For this review, use the dimensioned drawing (mm, ordinates from the lowest corner) and the shaded views. A direction names the side the tool comes from. Coordinates: 2 decimals unless noted, no trailing zeros. Order: outer loops, then holes, each group sorted by start corner. A loop starts at its lowest first (then second) coordinate and runs counter-clockwise, first axis right, second up. Notation, with made-up numbers: M 62.25,-4 L 88.25,-4 A12 cw 88.25,18 Z; hole C -36.5,-5.5 d1. An arc over 180 degrees is marked long. Use CSV: the item, a comma, the result in double quotes.
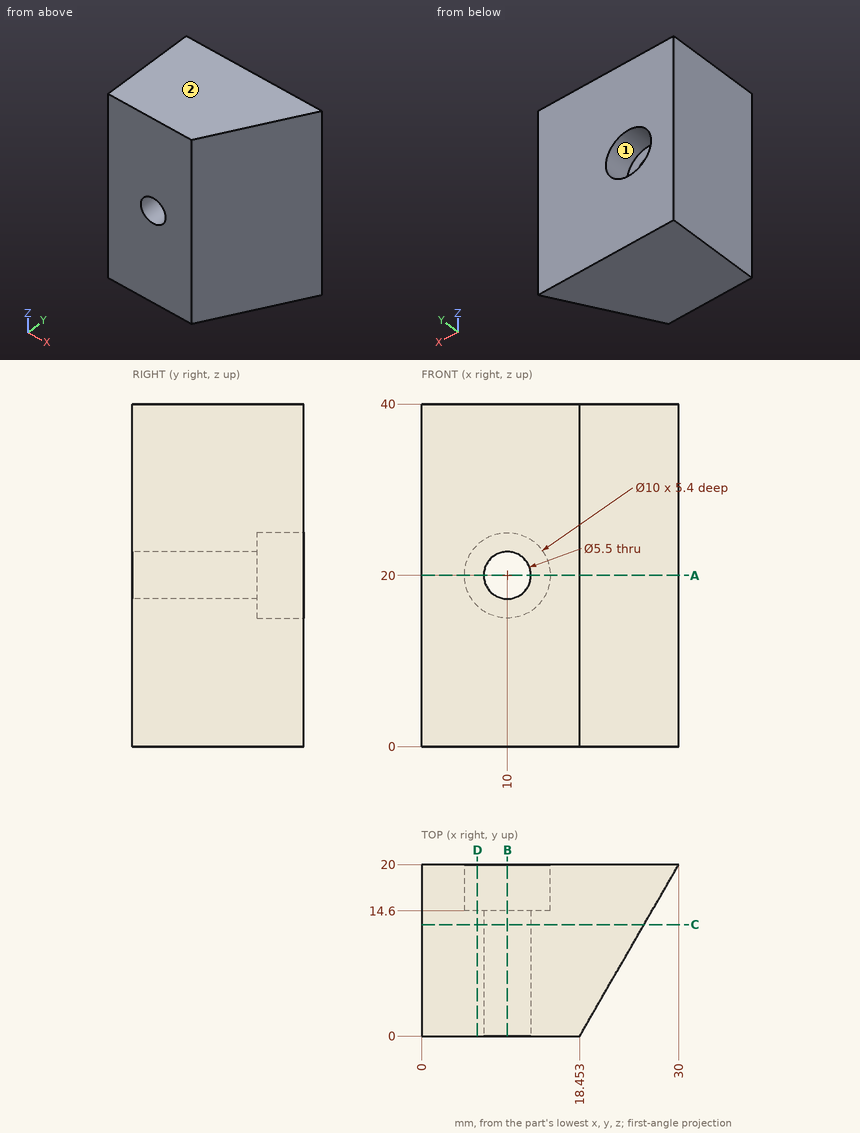
Item 1: Clearance check with flat-ended pins moving along their axes: pin 1 Ø3 at (y, z) = (8, 21.5) entering from +X; pin 2 Ø9 at (x, z) = (10, 20) entering from +Y. State where each tip first meets the part, or that it passes through.
Solutions:
pin 1,"x = 23.94"
pin 2,"y = 14.6"
Item 2: Add section C-C on y = 13. State the section outline as (x, z) points.
Solutions:
outline,"M 0,0 L 25.96,0 L 25.96,40 L 0,40 Z; hole C 10,20 d5.5"
Item 3: Add section D-D on x = 6.5. State the section outline as (y, z) points.
Solutions:
outline,"M 0,0 L 20,0 L 20,16.43 L 14.6,16.43 L 14.6,23.57 L 20,23.57 L 20,40 L 0,40 Z"
Item 4: To check wall thickness, follow line 1 along Z through (x, y) = (10, 16.65); line 2 along Z through (x, y) = (10, 10.25); line 3 along X through (y, z) = (8.5, 21.5). State the ranges of each line that lie inside material, in increasing order. Write a range as [from, to].
Solutions:
line 1,"[0, 15], [25, 40]"
line 2,"[0, 17.25], [22.75, 40]"
line 3,"[0, 7.7], [12.3, 23.36]"
Item 5: Add section B-B on x = 10. State the section outline as (y, z) points.
Solutions:
outline,"M 0,0 L 20,0 L 20,15 L 14.6,15 L 14.6,17.25 L 0,17.25 Z; M 0,22.75 L 14.6,22.75 L 14.6,25 L 20,25 L 20,40 L 0,40 Z"
Item 6: For the marked faces 1 and 2, list the 3-axis set-ups (+Z, -Z, +X, -X, +Y, -Y) from which the entire face can be reached by the end or side of a thin tool; tool diameter is ignored.
Solutions:
face 1,"+Y"
face 2,"+Z, +X, -X, +Y, -Y"
Item 7: Add section A-A on z = 20. State the section outline as (x, y) points, and give its area (3 significant figures).
Solutions:
outline,"M 0,0 L 7.25,0 L 7.25,14.6 L 5,14.6 L 5,20 L 0,20 Z; M 12.75,0 L 18.45,0 L 30,20 L 15,20 L 15,14.6 L 12.75,14.6 Z"
area,"350 mm^2"
